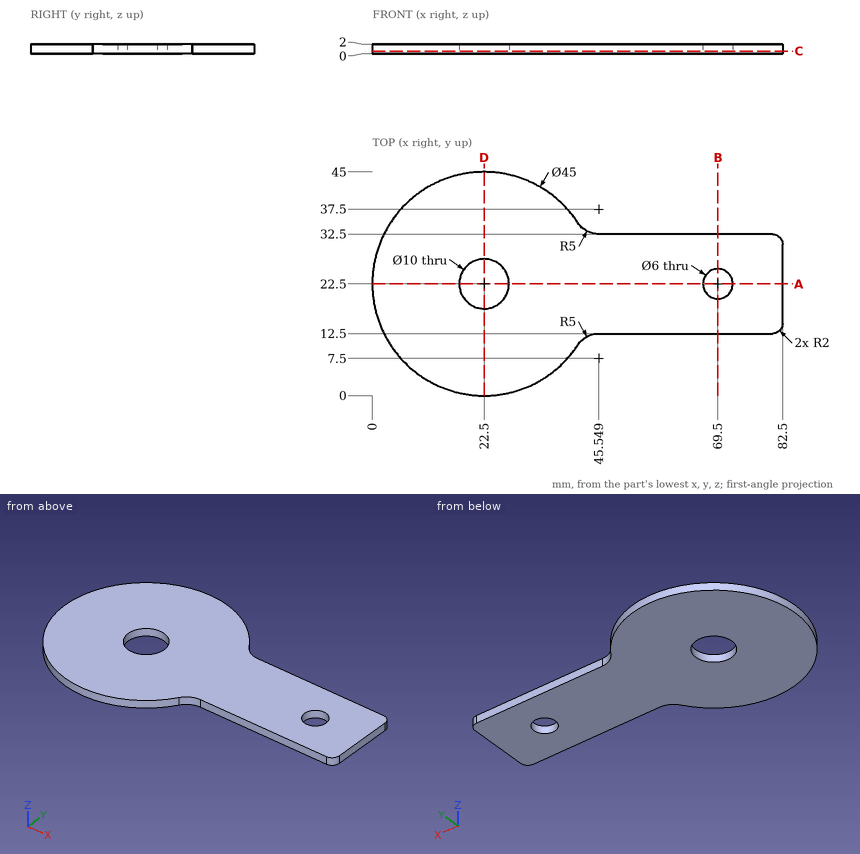
Source: three-view drawing plus pictorial views. Frame: mm from the lowest corner of the part. Give positions to 0.01 mm unless a question says otherwise; leave off trailing zeros. Loops run counter-clockwise (first coordinate to the right, second up) from the corner with the lowest first, then second, coordinate; pieces in that order, holes last.
1) Contact query for flat-ended pins moving along their axis: pin 1 (0.6 mm diameter, centred on x = 58.5, z = 0.5, fed in from -Y); pin 2 (1 mm diameter, centred on x = 70, z = 1.5, fed in from +Y). Output: stop coordinate, or through.
A:
pin 1: stops at y = 12.5
pin 2: stops at y = 32.5
2) Section query D-D on x = 22.5. Return the cut outline in (y, z), and give its area (3 significant figures).
A:
outline: (0, 0) - (17.5, 0) - (17.5, 2) - (0, 2) - close; (27.5, 0) - (45, 0) - (45, 2) - (27.5, 2) - close
area: 70.0 mm2
3) Section query B-B on x = 69.5. Return the cut outline in (y, z), and give its area (3 significant figures).
A:
outline: (12.5, 0) - (19.5, 0) - (19.5, 2) - (12.5, 2) - close; (25.5, 0) - (32.5, 0) - (32.5, 2) - (25.5, 2) - close
area: 28.0 mm2
4) Section query A-A on y = 22.5. Return the cut outline in (x, z), and give its area (3 significant figures).
A:
outline: (0, 0) - (17.5, 0) - (17.5, 2) - (0, 2) - close; (27.5, 0) - (66.5, 0) - (66.5, 2) - (27.5, 2) - close; (72.5, 0) - (82.5, 0) - (82.5, 2) - (72.5, 2) - close
area: 133 mm2
5) Line query: L1, parallel to X at y = 20.5, z = 1.95; L2, parallel to Y at x = 69.5, z = 1.5; L3, parallel to Y at x = 22.5, z = 0.55. Output: solid intervals per line, ascending.
A:
L1: x = 0.09 to 17.92, 27.08 to 67.26, 71.74 to 82.5
L2: y = 12.5 to 19.5, 25.5 to 32.5
L3: y = 0 to 17.5, 27.5 to 45
6) Section query C-C on z = 0.55. Return the cut outline in (x, y).
A:
outline: (41.36, 10.23) arc R5 cw to (45.55, 12.5) - (80.5, 12.5) arc R2 ccw to (82.5, 14.5) - (82.5, 30.5) arc R2 ccw to (80.5, 32.5) - (45.55, 32.5) arc R5 cw to (41.36, 34.77) arc R22.5 ccw (long way) to start; hole circle Ø10 at (22.5, 22.5); hole circle Ø6 at (69.5, 22.5)
